Geometry: final body of the model. Coordinates: model frame, mm. Face numbers are marked on the shaded views. Give positions to 0.01 mm unless a question says otherwise; leave off trailing zeros. Write each loop counter-clockwise with the first axis right and the second up, starting at its lowest first coordinate (ties: lowest second). Pieces come first, ordered by that corner, then holes. Notation, with made-up numbers: M 16.25,26.5 L 40.25,26.5 A22 cw 40.25,56.5 Z; hole C 30,-5 d9. An arc over 180 degrees is marked long. One line per question, with ' | ' between items.
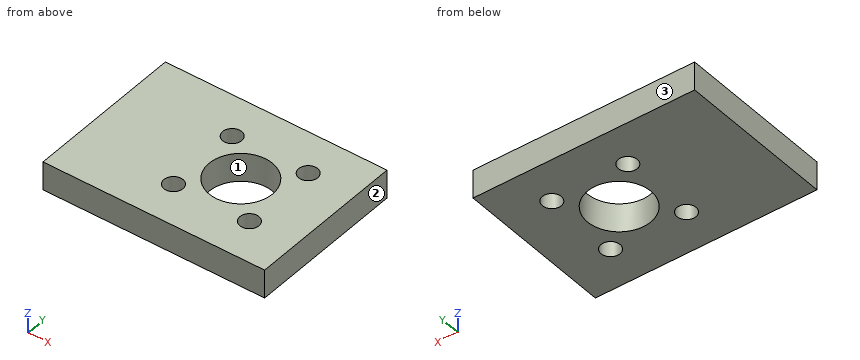
from build123d import *

# Parameters (mm, degrees)
F0_R     = 1.5
F0_R_2   = 5
F1_DEPTH = 4.5


with BuildPart() as f1:
    # F0 (on Top) → F1 (new body)
    with BuildSketch(Plane.XY):
        Polygon((-27.597585, 28.725847), (-62.592236, 28.725847), (-62.597585, 3.733337), (-27.597585, 3.725847), align=None)
        with Locations((-47.017195, 10.225847)):
            Circle(F0_R, mode=Mode.SUBTRACT)
        with Locations((-41.017195, 16.225847)):
            Circle(F0_R_2, mode=Mode.SUBTRACT)
        with Locations((-35.017195, 10.225847)):
            Circle(F0_R, mode=Mode.SUBTRACT)
        with Locations((-47.017195, 22.225847)):
            Circle(F0_R, mode=Mode.SUBTRACT)
        with Locations((-35.017195, 22.225847)):
            Circle(F0_R, mode=Mode.SUBTRACT)
    extrude(amount=F1_DEPTH)


solid = f1.part
(1) First-contact query: P1, Ø1.5, axis at x = -47, z = 2, coming from the -Y side; P2, Ø1.5, axis at y = 22, z = 4, coming from the -X side. Flat tips, straight axial feed; report the tip coordinate or a pass-through.
Working result:
P1: stops at y = 3.73 | P2: stops at x = -62.59
(2) Material intervals for L1, parallel to X at y = 22.25, z = 3.15; L2, parallel to X at y = 21.75, z = 2.7; L3, parallel to Y at x = -51.5, z = 4.1, sorted ascending. Write a range as [from, to].
Working result:
L1: x = [-62.59, -48.52], [-45.52, -36.52], [-33.52, -27.6] | L2: x = [-62.59, -48.44], [-45.59, -36.44], [-33.59, -27.6] | L3: y = [3.73, 28.73]
(3) Cut plane D-D, the plane x = -44. Return loops of the section in (y, z), then the cut area to 3 significant figures.
Working result:
outline: M 3.73,0 L 12.21,0 L 12.21,4.5 L 3.73,4.5 Z; M 20.24,0 L 28.73,0 L 28.73,4.5 L 20.24,4.5 Z | area: 76.4 mm^2
(4) Cut plane C-C, the plane z = 1.35. Return loops of the section in (x, y), then the cut area to 3 significant figures.
Working result:
outline: M -62.6,3.73 L -27.6,3.73 L -27.6,28.73 L -62.59,28.73 Z; hole C -47.02,10.23 d3; hole C -47.02,22.23 d3; hole C -41.02,16.23 d10; hole C -35.02,10.23 d3; hole C -35.02,22.23 d3 | area: 768 mm^2
(5) Cut plane A-A, the plane y = 17.5. Return loops of the section in (x, z), then the cut area to 3 significant figures.
Working result:
outline: M -62.59,0 L -45.85,0 L -45.85,4.5 L -62.59,4.5 Z; M -36.18,0 L -27.6,0 L -27.6,4.5 L -36.18,4.5 Z | area: 114 mm^2
(6) Draft query along Y for the marked faces 1, 2 and 3. Return one class per face: released by +Y, released by -Y, zero draft, split by the parting line, or undercut.
Working result:
face 1: undercut | face 2: zero draft | face 3: released by +Y
(7) Cut plane B-B, the plane x = -47.5. Return loops of the section in (y, z), then the cut area to 3 significant figures.
Working result:
outline: M 3.73,0 L 8.81,0 L 8.81,4.5 L 3.73,4.5 Z; M 11.65,0 L 20.81,0 L 20.81,4.5 L 11.65,4.5 Z; M 23.65,0 L 28.73,0 L 28.73,4.5 L 23.65,4.5 Z | area: 86.9 mm^2
